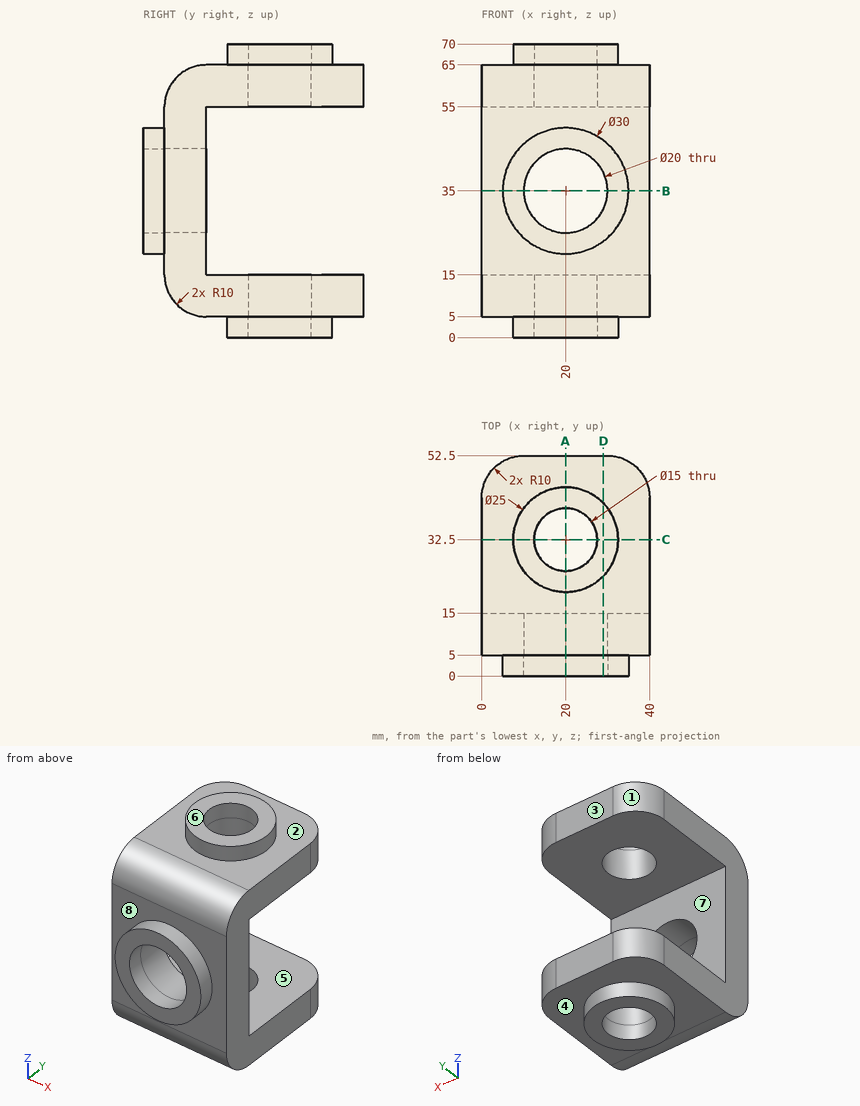
Part print with two shaded views. Sizes in mm from the minimum x, y, z corner. A direction names the side the tool comes from. Coordinates: 2 decimals unless noted, no trailing zeros. Write each loop counter-clockwise with the first axis right and the second up, starting at its lowest first coordinate (ties: lowest second). Pieces come first, ordered by that corner, then holes.
1. Drop flat-ended pins along their axis: pin 1 (5 mm diameter, centred on x = 6.5, z = 24, fed in from +Y); pin 2 (13.5 mm diameter, centred on x = 20, y = 32.5, fed in from -Z); pin 3 (8 mm diameter, centred on x = 24.5, y = 12, fed in from -Z); pin 4 (10 mm diameter, centred on x = 6, z = 50.5, fed in from +Y). Give the stop position or say it passes through.
Answer block:
pin 1: stops at y = 15
pin 2: passes through
pin 3: stops at z = 5
pin 4: stops at y = 52.33
2. 3-axis set-ups, long thin cutter, end or side, ignore diameter. For the marked faces 1, 2, 3, 4 and 5: which of +Z, -Z, +X, -X, +Y, -Y reach the whole face in a straight line?
Answer block:
face 1: +Z, -Z, -X, +Y
face 2: +Z
face 3: +Z, -Z, +X, -X, +Y
face 4: -Z
face 5: +X, -X, +Y
3. Band-saw the part on C-C, the plane y = 32.5. Give the cut face in (x, z), and give its area (3 significant figures).
Answer block:
outline: (0, 5) - (7.5, 5) - (7.5, 0) - (12.5, 0) - (12.5, 15) - (0, 15) - close; (0, 55) - (12.5, 55) - (12.5, 70) - (7.5, 70) - (7.5, 65) - (0, 65) - close; (27.5, 0) - (32.5, 0) - (32.5, 5) - (40, 5) - (40, 15) - (27.5, 15) - close; (27.5, 55) - (40, 55) - (40, 65) - (32.5, 65) - (32.5, 70) - (27.5, 70) - close
area: 600 mm2
4. Band-saw the part on D-D, the plane x = 29. Give the cut face in (y, z), and give its area (3 significant figures).
Answer block:
outline: (0, 23) - (5, 23) - (5, 15) arc R10 ccw to (15, 5) - (23.83, 5) - (23.83, 0) - (41.17, 0) - (41.17, 5) - (52.5, 5) - (52.5, 15) - (15, 15) - (15, 30.64) - (0, 30.64) - close; (0, 39.36) - (15, 39.36) - (15, 55) - (52.5, 55) - (52.5, 65) - (41.17, 65) - (41.17, 70) - (23.83, 70) - (23.83, 65) - (15, 65) arc R10 ccw to (5, 55) - (5, 47) - (0, 47) - close
area: 1,470 mm2
5. Drill centre lines: probe 1 along Z at (x, y) = (2.5, 33); probe 2 along Z at (x, y) = (20, 1); probe 3 along Y at (x, z) = (20, 2.65). Where is each one in solid material? Low to high.
Answer block:
probe 1: z = 5 to 15, 55 to 65
probe 2: z = 20 to 25, 45 to 50
probe 3: y = 20 to 25, 40 to 45
6. Pull direction Z, two halves, no side cores. Call the marked faces 6, 7 and 8: released by +Z, released by -Z, zero draft, split by the parting line, or undercut.
Answer block:
face 6: released by +Z
face 7: undercut
face 8: zero draft
7. Band-saw the part on A-A, the plane x = 20. Give the number of separate pieces and of enclosed holes in the cut face, and give its area (3 significant figures).
Answer block:
separate pieces: 4
enclosed holes: 0
area: 957 mm2
8. Band-saw the part on B-B, the plane z = 35. Give the cut face in (x, y).
Answer block:
outline: (0, 5) - (5, 5) - (5, 0) - (10, 0) - (10, 15) - (0, 15) - close; (30, 0) - (35, 0) - (35, 5) - (40, 5) - (40, 15) - (30, 15) - close
